Can you work these out from the drawing? Everything is in mm from the part's minimum corner. A direction names the side the tool comes from. Coordinates: 2 decimals unless noted, no trailing zeros. Loops run counter-clockwise (first coordinate to the right, second up) from the corner with the lowest first, then second, coordinate; pieces in that order, holes last.
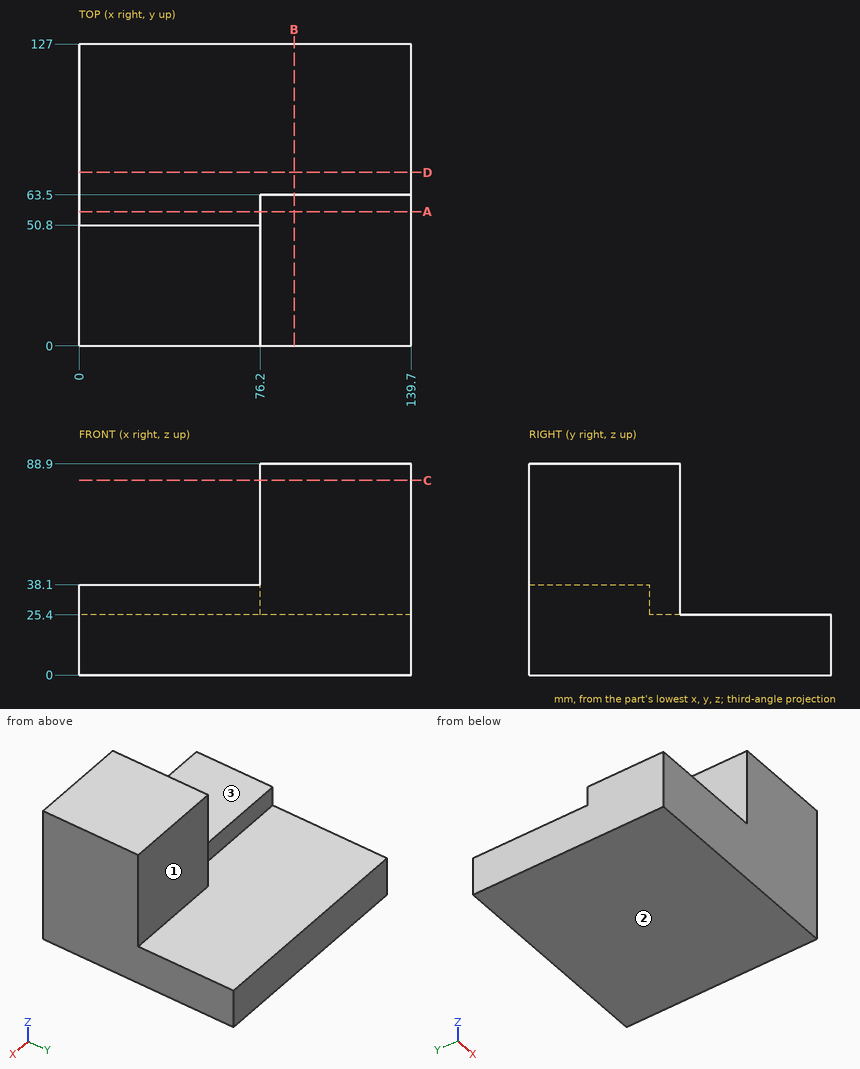
1) For the marked faces 1, 2 and 3, which set-ups out of +Z, -Z, +X, -X, +Y, -Y let a thin tool reach every point of the face, with its end or its side?
2) Will these pins go through, and if not, where does the flat tip stop? pin 1 (2 mm diameter, centred on x = 32, z = 29, fed in from -Y); pin 2 (10 mm diameter, centred on x = 71.5, z = 68.5, fed in from +Y); pin 3 (12 mm diameter, centred on y = 68, z = 76.5, fed in from -X); pin 4 (10 mm diameter, centred on x = 35.5, z = 33.5, fed in from +Y).
3) Imagine slicing it at A-A on y = 56.5. List the corners of the cut face in (x, z) for me.
4) If I drill on L1, parallel to Z at x = 62, y = 112; L2, parallel to Y at x = 101, z = 73.5; L3, parallel to Z at x = 72.5, y = 45, over which ranges is the centre line in solid material (lowest first)?
5) Imagine slicing it at D-D on y = 73. List the corners of the cut face in (x, z) for me, plus the area to 3 significant figures.
6) Imagine slicing it at C-C on z = 82. List the corners of the cut face in (x, y) for me, plus the area to 3 significant figures.
7) Imagine slicing it at B-B on x = 90.5. List the corners of the cut face in (y, z) for me, plus the area to 3 significant figures.
Solved:
1. face 1: +Z, +X, -X, +Y
1. face 2: -Z, +X, -X, +Y, -Y
1. face 3: +Z, -X, +Y, -Y
2. pin 1: stops at y = 0
2. pin 2: stops at y = 63.5
2. pin 3: stops at x = 76.2
2. pin 4: stops at y = 50.8
3. outline: (0, 0) - (139.7, 0) - (139.7, 88.9) - (76.2, 88.9) - (76.2, 25.4) - (0, 25.4) - close
4. L1: z = 0 to 25.4
4. L2: y = 0 to 63.5
4. L3: z = 0 to 38.1
5. outline: (0, 0) - (139.7, 0) - (139.7, 25.4) - (0, 25.4) - close
5. area: 3,550 mm2
6. outline: (76.2, 0) - (139.7, 0) - (139.7, 63.5) - (76.2, 63.5) - close
6. area: 4,030 mm2
7. outline: (0, 0) - (127, 0) - (127, 25.4) - (63.5, 25.4) - (63.5, 88.9) - (0, 88.9) - close
7. area: 7,260 mm2
